Verification items for the finished model (mm, model axes). Face numbers are marked on the shaded views. A direction names the side the tool comes from. Round coordinates to 2 decimals unless told otherwise and drop trailing zeros. Write each loop counter-clockwise with the first axis right and the second up, starting at its lowest first coordinate (ties: lowest second). Pieces come first, ordered by that corner, then holes. Notation, with made-up numbers: (-9.5, -17) - (31.5, -17) arc R19 cw to (31.5, 19) - close; hole circle Ø2 at (80.25, 27). An arc over 180 degrees is marked (long way). Answer as a JSON object with one key per item and string values. Group by question number.
1) Section check D-D (x = 13). Enter the section's corners in (y, z).
2) Section check B-B (x = 19.25). Enter the section's corners in (y, z) (3 decimals), then the cut area to 3 significant figures.
3) Set-up check for the marked faces 1, 2 and 3: record each of +Z, -Z, +X, -X, +Y, -Y from which the full face is reachable in a straight line by a thin tool's end or side.
4) Thickness scan on line 1 (X direction, y = -8.5, z = 4.5); line 2 (X direction, y = 9.5, z = 8.75); line 3 (Z direction, x = 21.5, y = -2). Record the ranges inside material, lowest first.
5) Section check C-C (y = -3). Enter the section's corners in (x, z) (3 decimals), then the cut area to 3 significant figures.
6) Section check A-A (z = 11.75). Enter the section's corners in (x, y) (3 decimals), then the cut area to 3 significant figures.
7) Mould release check, pull along X, two halves, no side actions. Record for the marked faces 4, 5 and 6: +X half, -X half, draft (parallel to the pull), parting line (faces both ways), or undercut.
8) Go/stop test with flat-tipped pins: pin 1 Ø5 at (x, y) = (19, 0.5) entering from +Z; pin 2 Ø4 at (x, z) = (6.5, 4.5) entering from -Y; pin 3 Ø5 at (y, z) = (22, 3) entering from -X. Record where each tip stops, or that it passes through.
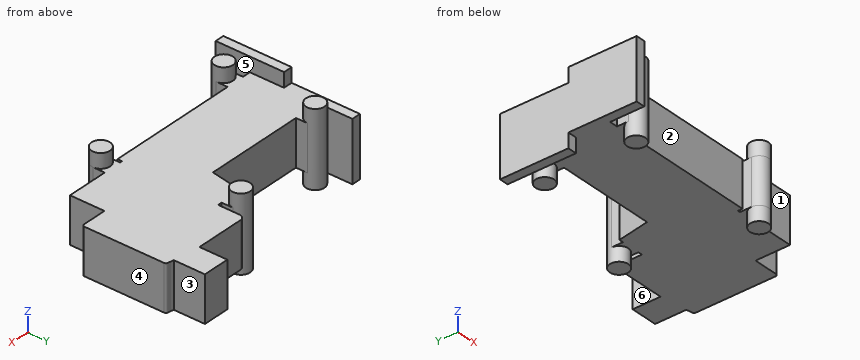
```python
from build123d import *

# Parameters (mm, degrees)
SKETCH1_W                = 25.4
SKETCH1_H                = 15
BOSS_EXTRUDE1_DEPTH      = 10
BOSS_EXTRUDE2_DEPTH      = 10
SKETCH3_W                = 3.175
SKETCH3_H                = 14.99375
BOSS_EXTRUDE3_DEPTH      = 2
BOSS_EXTRUDE6_DEPTH      = 10
BOSS_EXTRUDE7_DEPTH      = 3.175
BOSS_EXTRUDE7_DEPTH_BACK = 13.175
SKETCH7_R                = 2.032


with BuildPart() as part:
    # Sketch1 → Boss-Extrude1 (new body)
    with BuildSketch(Plane.XY):
        Rectangle(SKETCH1_W, SKETCH1_H)
    extrude(amount=BOSS_EXTRUDE1_DEPTH)

    # Sketch2 → Boss-Extrude2 (add)
    with BuildSketch(Plane.XY.offset(10)):
        with BuildLine():
            Line((40.1, 19.759426681), (40.970013246, 19.606019872))
            Line((40.970013246, 19.606019872), (41.386824089, 19.532524875))
            ThreePointArc((41.386824089, 19.532524875), (41.683022222, 19.361514803), (41.8, 19.040120998))
            Line((41.8, 19.040120998), (41.8, 1.55))
            ThreePointArc((41.8, 1.55), (41.653553391, 1.196446609), (41.3, 1.05))
            Line((41.3, 1.05), (40.883189158, 1.05))
            Line((40.883189158, 1.05), (35.9, 1.05))
            Line((35.9, 1.05), (35.9, -2.35))
            Line((35.9, -2.35), (35.9, -6.5))
            Line((35.9, -6.5), (34.9, -6.5))
            Line((34.9, -6.5), (22.2, -6.5))
            Line((22.2, -6.5), (22.2, -7.5))
            Line((22.2, -7.5), (9.4, -7.5))
            Line((9.4, -7.5), (9.4, 7.5))
            Line((9.4, 7.5), (15.048, 7.5))
            Line((15.048, 7.5), (16.3, 14.6))
            Line((16.3, 14.6), (22.2, 14.6))
            Line((22.2, 14.6), (22.2, 19.3))
            ThreePointArc((22.2, 19.3), (22.551471863, 20.148528137), (23.4, 20.5))
            Line((23.4, 20.5), (34.2, 20.5))
            Line((34.2, 20.5), (34.2, 26.6))
            Line((34.2, 26.6), (40.1, 26.6))
            Line((40.1, 26.6), (40.1, 19.759426681))
        make_face()
        Polygon((-14.7, 14.2), (-14.7, 14.99375), (-12.7, 14.99375), (-12.7, 14.2), (-12.7, 12.710514427), (-12.7, 7.5), (-12.7, 0), (-12.7, -10.069090909), (-12.7, -14.2), (-12.7, -14.99375), (-14.7, -14.99375), (-14.7, -14.2), (-14.7, -10.069090909), (-14.7, 0), (-14.7, 7.5), (-14.7, 11), align=None)
    extrude(amount=-BOSS_EXTRUDE2_DEPTH)

    # Sketch3 → Boss-Extrude3 (add)
    with BuildSketch(Plane.ZY.offset(14.7)):
        with Locations((-1.5875, 7.496875)):
            Rectangle(SKETCH3_W, SKETCH3_H)
        with Locations((11.5875, -7.496875)):
            Rectangle(SKETCH3_W, SKETCH3_H)
    extrude(amount=-BOSS_EXTRUDE3_DEPTH)

    # Sketch6 → Boss-Extrude6 (add)
    with BuildSketch(Plane.XY.offset(10)):
        with BuildLine():
            Line((-10.887, 7.5), (-10.887, 10.04))
            ThreePointArc((-10.887, 10.04), (-8.855, 12.072), (-6.823, 10.04))
            Line((-6.823, 10.04), (-6.823, 7.5))
            ThreePointArc((-6.823, 7.5), (-8.855, 5.468), (-10.887, 7.5))
        make_face()
        with BuildLine():
            Line((-10.887, -7.5), (-10.887, -10.04))
            ThreePointArc((-10.887, -10.04), (-8.855, -12.072), (-6.823, -10.04))
            Line((-6.823, -10.04), (-6.823, -7.5))
            ThreePointArc((-6.823, -7.5), (-8.855, -5.468), (-10.887, -7.5))
        make_face()
        with BuildLine():
            Line((17.218, 14.6), (17.218, 17.14))
            ThreePointArc((17.218, 17.14), (19.25, 19.172), (21.282, 17.14))
            Line((21.282, 17.14), (21.282, 14.6))
            ThreePointArc((21.282, 14.6), (19.25, 12.568), (17.218, 14.6))
        make_face()
        with BuildLine():
            Line((26.772, -6.5), (26.772, -9.04))
            ThreePointArc((26.772, -9.04), (24.74, -11.072), (22.708, -9.04))
            Line((22.708, -9.04), (22.708, -6.5))
            ThreePointArc((22.708, -6.5), (24.74, -4.468), (26.772, -6.5))
        make_face()
    extrude(amount=-BOSS_EXTRUDE6_DEPTH)

    # Sketch7 → Boss-Extrude7 (add, two sides: drawn at the far end of the back side and taken through both)
    with BuildSketch(Plane(origin=(0, 0, 0), x_dir=(-1, 0, 0), z_dir=(0, 0, -1)).offset(-BOSS_EXTRUDE7_DEPTH_BACK)):
        with Locations((-19.25, 17.14)):
            Circle(SKETCH7_R)
        with Locations((-24.74, -9.04)):
            Circle(SKETCH7_R)
        with Locations((8.855, -10.04)):
            Circle(SKETCH7_R)
        with Locations((8.855, 10.04)):
            Circle(SKETCH7_R)
    extrude(amount=BOSS_EXTRUDE7_DEPTH + BOSS_EXTRUDE7_DEPTH_BACK)


solid = part.part
```
Returned:
{
 "1": {"outline": "(-7.5, 0) - (7.5, 0) - (7.5, 10) - (-7.5, 10) - close"},
 "2": {"outline": "(-7.5, 0) - (15.108, 0) - (15.108, -3.175) - (19.172, -3.175) - (19.172, 13.175) - (15.108, 13.175) - (15.108, 10) - (-7.5, 10) - close", "area": "293 mm2"},
 "3": {"face 1": "+Z, -Z, +X, -Y", "face 2": "+Z, -Z, -Y", "face 3": "+Z, -Z, +X, +Y"},
 "4": {"line 1": "-14.7 to -12.7, -10.89 to -6.82, 22.71 to 26.77", "line 2": "-14.7 to -12.7, -10.89 to -6.82, 15.4 to 41.8", "line 3": "0 to 10"},
 "5": {"outline": "(-14.7, 0) - (35.9, 0) - (35.9, 10) - (-12.7, 10) - (-12.7, 13.175) - (-14.7, 13.175) - close", "area": "512 mm2"},
 "6": {"outline": "(-14.7, -14.994) - (-12.7, -14.994) - (-12.7, 0) - (-14.7, 0) - close; circle Ø4.064 at (-8.855, -10.04); circle Ø4.064 at (-8.855, 10.04); circle Ø4.064 at (19.25, 17.14); circle Ø4.064 at (24.74, -9.04)", "area": "81.9 mm2"},
 "7": {"face 4": "+X half", "face 5": "undercut", "face 6": "-X half"},
 "8": {"pin 1": "z = 10", "pin 2": "y = -7.5", "pin 3": "x = 22.22"}
}
